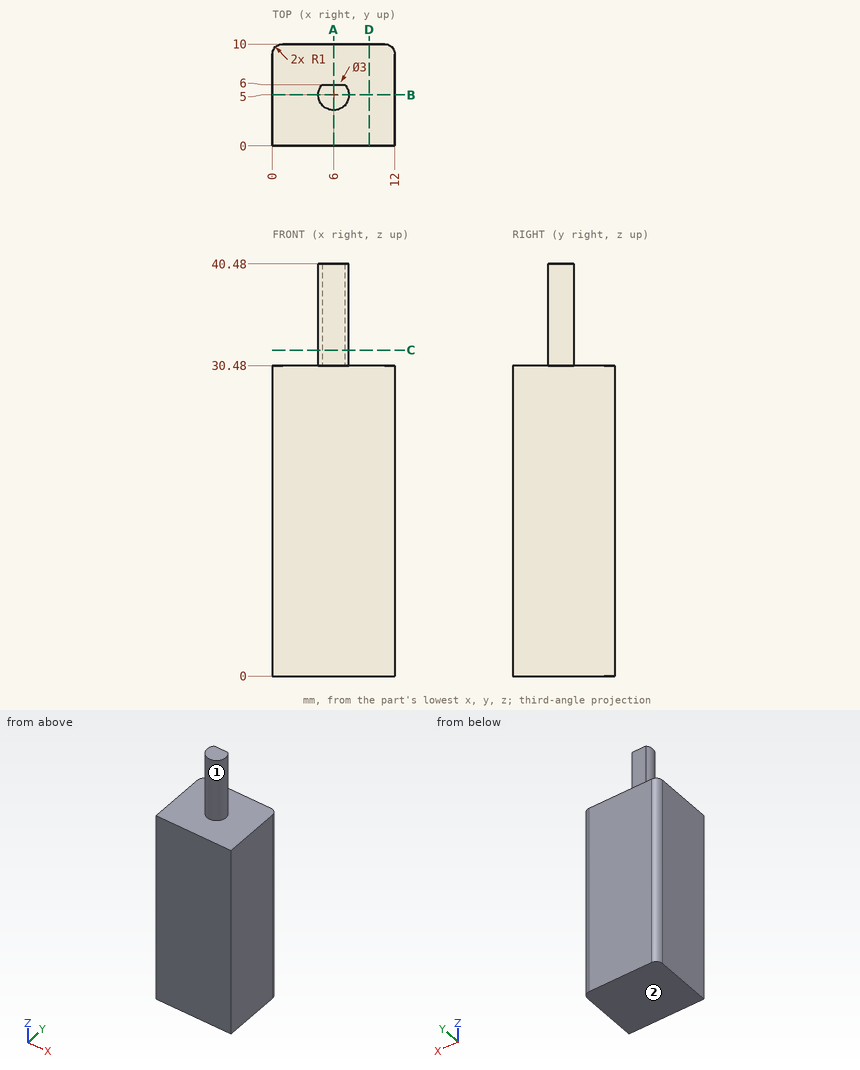
The drawing under review shows one solid part. Ordinate dimensions are in mm from its lowest x, y, z. A direction names the side the tool comes from. Round coordinates to 2 decimals unless told otherwise and drop trailing zeros. Write each loop counter-clockwise with the first axis right and the second up, starting at its lowest first coordinate (ties: lowest second). Pieces come first, ordered by that corner, then holes. Notation, with made-up numbers: (14, 25.5) -> (73, 25.5) arc R13 ccw to (73, 47.5) -> close; hole circle Ø1 at (-23, -14.75). An arc over 180 degrees is marked (long way). One line per question, with ' | ' between items.
(1) Take a section at C-C, the plane z = 32. State the section outline as (x, y) points.
Result sheet:
outline: (4.88, 6) arc R1.5 ccw (long way) to (7.12, 6) -> close
(2) Wall thickness on line 1 (Z direction, x = 11.5, y = 2); line 2 (Y direction, x = 0.5, z = 3.5); line 3 (Y direction, x = 6.75, z = 36): over which ranges is each line inside the solid? List them lowest first. Write a range as [from, to].
Result sheet:
line 1: [0, 30.48] | line 2: [0, 9.87] | line 3: [3.7, 6]
(3) Take a section at B-B, the plane y = 5. State the section outline as (x, z) points.
Result sheet:
outline: (0, 0) -> (12, 0) -> (12, 30.48) -> (7.5, 30.48) -> (7.5, 40.48) -> (4.5, 40.48) -> (4.5, 30.48) -> (0, 30.48) -> close
(4) Machinability: for the marked faces 1 and 2, which of the approach directions +Z, -Z, +X, -X, +Y, -Y give a long, thin tool a straight path to every point of the face, cutting with its end or side? Answer none if there is none.
Result sheet:
face 1: +Z | face 2: -Z, +X, -X, +Y, -Y
(5) Insertion check: P1, Ø2.5, axis at x = 5.5, z = 37.5, coming from the +Y side. The pin has a flat end and moves straight along its axis. Give the tip position at first contact, or say it passes through.
Result sheet:
P1: y = 6
(6) Take a section at A-A, the plane x = 6. State the section outline as (y, z) points.
Result sheet:
outline: (0, 0) -> (10, 0) -> (10, 30.48) -> (6, 30.48) -> (6, 40.48) -> (3.5, 40.48) -> (3.5, 30.48) -> (0, 30.48) -> close
(7) Take a section at D-D, the plane x = 9.5. State the section outline as (y, z) points, and give its area (3 significant figures).
Result sheet:
outline: (0, 0) -> (10, 0) -> (10, 30.48) -> (0, 30.48) -> close | area: 305 mm2
